Design review of the part built by this model. Coordinates are the model's own, in mm. Face numbers are marked on the shaded views. Coordinates: 2 decimals unless noted, no trailing zeros. Loops run counter-clockwise (first coordinate to the right, second up) from the corner with the lowest first, then second, coordinate; pieces in that order, holes last. Notation, with made-up numbers: (69, 0) -> (99, 0) arc R18 ccw to (99, 25) -> close; hole circle Ø1 at (21.5, 10). An arc over 180 degrees is marked (long way). Answer as a JSON object with one key per item and string values.
```python
from build123d import *

# Parameters (mm, degrees)
BASIS_BLECH1_DEPTH              = 57.5
SCHNITT_LINEAR_AUSTRAGEN1_REACH = 68.785
SKIZZE6_R                       = 4
SKIZZE6_R_2                     = 1.2
SCHNITT_LINEAR_AUSTRAGEN2_REACH = 68.785
SKIZZE7_R                       = 1.65


# Sheet-metal steps are written as plain solids
with BuildPart() as part:
    # Skizze1 → Basis-Blech1 (new, symmetric)
    with BuildSketch(Plane(origin=(0, 0, 0), x_dir=(0, 0, -1), z_dir=(1, 0, 0))):
        with BuildLine():
            Line((-10.5, 25), (-10.5, 0.2))
            ThreePointArc((-10.5, 0.2), (-10.441421356, 0.058578644), (-10.3, 0))
            Line((-10.3, 0), (10.3, 0))
            ThreePointArc((10.3, 0), (10.441421356, 0.058578644), (10.5, 0.2))
            Line((10.5, 0.2), (10.5, 19))
            Line((10.5, 19), (11.5, 19))
            Line((11.5, 19), (11.5, 0.2))
            ThreePointArc((11.5, 0.2), (11.148528137, -0.648528137), (10.3, -1))
            Line((10.3, -1), (-10.3, -1))
            ThreePointArc((-10.3, -1), (-11.148528137, -0.648528137), (-11.5, 0.2))
            Line((-11.5, 0.2), (-11.5, 25))
            Line((-11.5, 25), (-10.5, 25))
        make_face()
    extrude(amount=BASIS_BLECH1_DEPTH, both=True)

    # Skizze6 → Schnitt-Linear austragen1 (cut, up to next)
    with BuildSketch(Plane.XY.offset(11.5), mode=Mode.PRIVATE) as schnitt_linear_austragen1_sk1:
        with Locations((-40, 12)):
            Circle(SKIZZE6_R)
    schnitt_linear_austragen1_tool1 = extrude(schnitt_linear_austragen1_sk1.sketch, amount=-SCHNITT_LINEAR_AUSTRAGEN1_REACH, mode=Mode.PRIVATE) & part.part
    # Skizze6 → Schnitt-Linear austragen1 (cut, up to next)
    with BuildSketch(Plane.XY.offset(11.5), mode=Mode.PRIVATE) as schnitt_linear_austragen1_sk2:
        with Locations((-53, 15)):
            Circle(SKIZZE6_R_2)
    schnitt_linear_austragen1_tool2 = extrude(schnitt_linear_austragen1_sk2.sketch, amount=-SCHNITT_LINEAR_AUSTRAGEN1_REACH, mode=Mode.PRIVATE) & part.part
    # Skizze6 → Schnitt-Linear austragen1 (cut, up to next)
    with BuildSketch(Plane.XY.offset(11.5), mode=Mode.PRIVATE) as schnitt_linear_austragen1_sk3:
        with Locations((-53, 3)):
            Circle(SKIZZE6_R_2)
    schnitt_linear_austragen1_tool3 = extrude(schnitt_linear_austragen1_sk3.sketch, amount=-SCHNITT_LINEAR_AUSTRAGEN1_REACH, mode=Mode.PRIVATE) & part.part
    # Skizze6 → Schnitt-Linear austragen1 (cut, up to next)
    with BuildSketch(Plane.XY.offset(11.5), mode=Mode.PRIVATE) as schnitt_linear_austragen1_sk4:
        with Locations((-27, 15)):
            Circle(SKIZZE6_R_2)
    schnitt_linear_austragen1_tool4 = extrude(schnitt_linear_austragen1_sk4.sketch, amount=-SCHNITT_LINEAR_AUSTRAGEN1_REACH, mode=Mode.PRIVATE) & part.part
    # Skizze6 → Schnitt-Linear austragen1 (cut, up to next)
    with BuildSketch(Plane.XY.offset(11.5), mode=Mode.PRIVATE) as schnitt_linear_austragen1_sk5:
        with Locations((-27, 3)):
            Circle(SKIZZE6_R_2)
    schnitt_linear_austragen1_tool5 = extrude(schnitt_linear_austragen1_sk5.sketch, amount=-SCHNITT_LINEAR_AUSTRAGEN1_REACH, mode=Mode.PRIVATE) & part.part
    # Skizze6 → Schnitt-Linear austragen1 (cut, up to next)
    with BuildSketch(Plane.XY.offset(11.5), mode=Mode.PRIVATE) as schnitt_linear_austragen1_sk6:
        with Locations(Location((53, 3, 0), (0, 0, 90))):
            Circle(SKIZZE6_R_2)
    schnitt_linear_austragen1_tool6 = extrude(schnitt_linear_austragen1_sk6.sketch, amount=-SCHNITT_LINEAR_AUSTRAGEN1_REACH, mode=Mode.PRIVATE) & part.part
    # Skizze6 → Schnitt-Linear austragen1 (cut, up to next)
    with BuildSketch(Plane.XY.offset(11.5), mode=Mode.PRIVATE) as schnitt_linear_austragen1_sk7:
        with Locations(Location((27, 3, 0), (0, 0, 90))):
            Circle(SKIZZE6_R_2)
    schnitt_linear_austragen1_tool7 = extrude(schnitt_linear_austragen1_sk7.sketch, amount=-SCHNITT_LINEAR_AUSTRAGEN1_REACH, mode=Mode.PRIVATE) & part.part
    # Skizze6 → Schnitt-Linear austragen1 (cut, up to next)
    with BuildSketch(Plane.XY.offset(11.5), mode=Mode.PRIVATE) as schnitt_linear_austragen1_sk8:
        with Locations(Location((27, 15, 0), (0, 0, 90))):
            Circle(SKIZZE6_R_2)
    schnitt_linear_austragen1_tool8 = extrude(schnitt_linear_austragen1_sk8.sketch, amount=-SCHNITT_LINEAR_AUSTRAGEN1_REACH, mode=Mode.PRIVATE) & part.part
    # Skizze6 → Schnitt-Linear austragen1 (cut, up to next)
    with BuildSketch(Plane.XY.offset(11.5), mode=Mode.PRIVATE) as schnitt_linear_austragen1_sk9:
        with Locations(Location((40, 12, 0), (0, 0, 90))):
            Circle(SKIZZE6_R)
    schnitt_linear_austragen1_tool9 = extrude(schnitt_linear_austragen1_sk9.sketch, amount=-SCHNITT_LINEAR_AUSTRAGEN1_REACH, mode=Mode.PRIVATE) & part.part
    # Skizze6 → Schnitt-Linear austragen1 (cut, up to next)
    with BuildSketch(Plane.XY.offset(11.5), mode=Mode.PRIVATE) as schnitt_linear_austragen1_sk10:
        with Locations(Location((53, 15, 0), (0, 0, 90))):
            Circle(SKIZZE6_R_2)
    schnitt_linear_austragen1_tool10 = extrude(schnitt_linear_austragen1_sk10.sketch, amount=-SCHNITT_LINEAR_AUSTRAGEN1_REACH, mode=Mode.PRIVATE) & part.part
    # Skizze6 → Schnitt-Linear austragen1 (cut, up to next)
    with BuildSketch(Plane.XY.offset(11.5), mode=Mode.PRIVATE) as schnitt_linear_austragen1_sk11:
        with BuildLine():
            Line((-20, 16), (-10, 16))
            ThreePointArc((-10, 16), (-6, 12), (-10, 8))
            Line((-10, 8), (-20, 8))
            ThreePointArc((-20, 8), (-24, 12), (-20, 16))
        make_face()
    schnitt_linear_austragen1_tool11 = extrude(schnitt_linear_austragen1_sk11.sketch, amount=-SCHNITT_LINEAR_AUSTRAGEN1_REACH, mode=Mode.PRIVATE) & part.part
    # Skizze6 → Schnitt-Linear austragen1 (cut, up to next)
    with BuildSketch(Plane.XY.offset(11.5), mode=Mode.PRIVATE) as schnitt_linear_austragen1_sk12:
        with BuildLine():
            Line((20, 16), (10, 16))
            ThreePointArc((10, 16), (6, 12), (10, 8))
            Line((10, 8), (20, 8))
            ThreePointArc((20, 8), (24, 12), (20, 16))
        make_face()
    schnitt_linear_austragen1_tool12 = extrude(schnitt_linear_austragen1_sk12.sketch, amount=-SCHNITT_LINEAR_AUSTRAGEN1_REACH, mode=Mode.PRIVATE) & part.part
    add(schnitt_linear_austragen1_tool1.solids().sort_by_distance((-40, 12, 11.5))[0], mode=Mode.SUBTRACT)
    add(schnitt_linear_austragen1_tool2.solids().sort_by_distance((-53, 15, 11.5))[0], mode=Mode.SUBTRACT)
    add(schnitt_linear_austragen1_tool3.solids().sort_by_distance((-53, 3, 11.5))[0], mode=Mode.SUBTRACT)
    add(schnitt_linear_austragen1_tool4.solids().sort_by_distance((-27, 15, 11.5))[0], mode=Mode.SUBTRACT)
    add(schnitt_linear_austragen1_tool5.solids().sort_by_distance((-27, 3, 11.5))[0], mode=Mode.SUBTRACT)
    add(schnitt_linear_austragen1_tool6.solids().sort_by_distance((53, 3, 11.5))[0], mode=Mode.SUBTRACT)
    add(schnitt_linear_austragen1_tool7.solids().sort_by_distance((27, 3, 11.5))[0], mode=Mode.SUBTRACT)
    add(schnitt_linear_austragen1_tool8.solids().sort_by_distance((27, 15, 11.5))[0], mode=Mode.SUBTRACT)
    add(schnitt_linear_austragen1_tool9.solids().sort_by_distance((40, 12, 11.5))[0], mode=Mode.SUBTRACT)
    add(schnitt_linear_austragen1_tool10.solids().sort_by_distance((53, 15, 11.5))[0], mode=Mode.SUBTRACT)
    add(schnitt_linear_austragen1_tool11.solids().sort_by_distance((-15, 12, 11.5))[0], mode=Mode.SUBTRACT)
    add(schnitt_linear_austragen1_tool12.solids().sort_by_distance((15, 12, 11.5))[0], mode=Mode.SUBTRACT)

    # Skizze7 → Schnitt-Linear austragen2 (cut, up to next)
    with BuildSketch(Plane(origin=(0, 0, -11.5), x_dir=(-1, 0, 0), z_dir=(0, 0, -1)), mode=Mode.PRIVATE) as schnitt_linear_austragen2_sk1:
        with Locations(Location((-40, 11.5, 0), (0, 0, 90))):
            Circle(SKIZZE7_R)
    schnitt_linear_austragen2_tool1 = extrude(schnitt_linear_austragen2_sk1.sketch, amount=-SCHNITT_LINEAR_AUSTRAGEN2_REACH, mode=Mode.PRIVATE) & part.part
    # Skizze7 → Schnitt-Linear austragen2 (cut, up to next)
    with BuildSketch(Plane(origin=(0, 0, -11.5), x_dir=(-1, 0, 0), z_dir=(0, 0, -1)), mode=Mode.PRIVATE) as schnitt_linear_austragen2_sk2:
        with Locations(Location((-20, 11.5, 0), (0, 0, 90))):
            Circle(SKIZZE7_R)
    schnitt_linear_austragen2_tool2 = extrude(schnitt_linear_austragen2_sk2.sketch, amount=-SCHNITT_LINEAR_AUSTRAGEN2_REACH, mode=Mode.PRIVATE) & part.part
    # Skizze7 → Schnitt-Linear austragen2 (cut, up to next)
    with BuildSketch(Plane(origin=(0, 0, -11.5), x_dir=(-1, 0, 0), z_dir=(0, 0, -1)), mode=Mode.PRIVATE) as schnitt_linear_austragen2_sk3:
        with Locations(Location((-10, 11.5, 0), (0, 0, 90))):
            Circle(SKIZZE7_R)
    schnitt_linear_austragen2_tool3 = extrude(schnitt_linear_austragen2_sk3.sketch, amount=-SCHNITT_LINEAR_AUSTRAGEN2_REACH, mode=Mode.PRIVATE) & part.part
    # Skizze7 → Schnitt-Linear austragen2 (cut, up to next)
    with BuildSketch(Plane(origin=(0, 0, -11.5), x_dir=(-1, 0, 0), z_dir=(0, 0, -1)), mode=Mode.PRIVATE) as schnitt_linear_austragen2_sk4:
        with Locations(Location((10, 11.5, 0), (0, 0, 90))):
            Circle(SKIZZE7_R)
    schnitt_linear_austragen2_tool4 = extrude(schnitt_linear_austragen2_sk4.sketch, amount=-SCHNITT_LINEAR_AUSTRAGEN2_REACH, mode=Mode.PRIVATE) & part.part
    # Skizze7 → Schnitt-Linear austragen2 (cut, up to next)
    with BuildSketch(Plane(origin=(0, 0, -11.5), x_dir=(-1, 0, 0), z_dir=(0, 0, -1)), mode=Mode.PRIVATE) as schnitt_linear_austragen2_sk5:
        with Locations(Location((20, 11.5, 0), (0, 0, 90))):
            Circle(SKIZZE7_R)
    schnitt_linear_austragen2_tool5 = extrude(schnitt_linear_austragen2_sk5.sketch, amount=-SCHNITT_LINEAR_AUSTRAGEN2_REACH, mode=Mode.PRIVATE) & part.part
    # Skizze7 → Schnitt-Linear austragen2 (cut, up to next)
    with BuildSketch(Plane(origin=(0, 0, -11.5), x_dir=(-1, 0, 0), z_dir=(0, 0, -1)), mode=Mode.PRIVATE) as schnitt_linear_austragen2_sk6:
        with Locations(Location((40, 11.5, 0), (0, 0, 90))):
            Circle(SKIZZE7_R)
    schnitt_linear_austragen2_tool6 = extrude(schnitt_linear_austragen2_sk6.sketch, amount=-SCHNITT_LINEAR_AUSTRAGEN2_REACH, mode=Mode.PRIVATE) & part.part
    add(schnitt_linear_austragen2_tool1.solids().sort_by_distance((40, 11.5, -11.5))[0], mode=Mode.SUBTRACT)
    add(schnitt_linear_austragen2_tool2.solids().sort_by_distance((20, 11.5, -11.5))[0], mode=Mode.SUBTRACT)
    add(schnitt_linear_austragen2_tool3.solids().sort_by_distance((10, 11.5, -11.5))[0], mode=Mode.SUBTRACT)
    add(schnitt_linear_austragen2_tool4.solids().sort_by_distance((-10, 11.5, -11.5))[0], mode=Mode.SUBTRACT)
    add(schnitt_linear_austragen2_tool5.solids().sort_by_distance((-20, 11.5, -11.5))[0], mode=Mode.SUBTRACT)
    add(schnitt_linear_austragen2_tool6.solids().sort_by_distance((-40, 11.5, -11.5))[0], mode=Mode.SUBTRACT)


solid = part.part
```
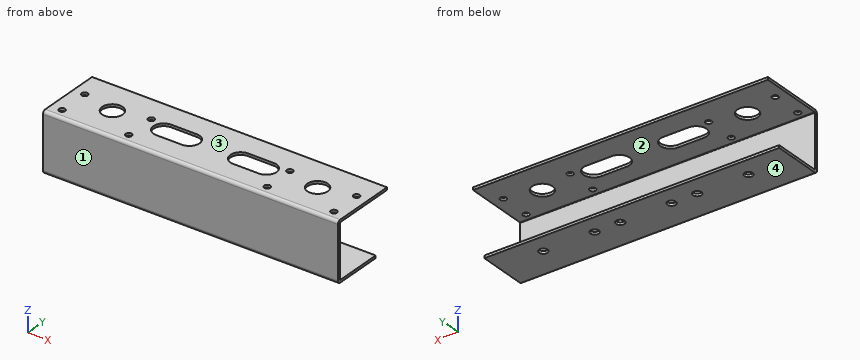
1) Wall thickness on probe 1 along Z at (x, y) = (29, 7.5); probe 2 along Y at (x, z) = (53, 11.2); probe 3 along Z at (x, y) = (9, 23.75): over which ranges is each line inside the solid? List them lowest first.
Completed:
{"probe 1": "-11.5 to -10.5, 10.5 to 11.5", "probe 2": "-0.59 to 1.8, 4.2 to 13.8, 16.2 to 25", "probe 3": "10.5 to 11.5"}
2) Add section D-D, the plane y = 21.25. Give the boundary of the cut face in (x, z).
Completed:
{"outline": "(-57.5, 10.5) -> (57.5, 10.5) -> (57.5, 11.5) -> (-57.5, 11.5) -> close"}
3) Add section B-B, the plane y = 3. Give the boundary of the cut face in (x, z).
Completed:
{"outline": "(-57.5, -11.5) -> (57.5, -11.5) -> (57.5, -10.5) -> (-57.5, -10.5) -> close; (-57.5, 10.5) -> (-54.2, 10.5) -> (-54.2, 11.5) -> (-57.5, 11.5) -> close; (-51.8, 10.5) -> (-28.2, 10.5) -> (-28.2, 11.5) -> (-51.8, 11.5) -> close; (-25.8, 10.5) -> (25.8, 10.5) -> (25.8, 11.5) -> (-25.8, 11.5) -> close; (28.2, 10.5) -> (51.8, 10.5) -> (51.8, 11.5) -> (28.2, 11.5) -> close; (54.2, 10.5) -> (57.5, 10.5) -> (57.5, 11.5) -> (54.2, 11.5) -> close"}
4) The part is to be moulded in two halves that separate along Z. For the marked faces 1, 2, 3 and 4, say which applies: pulls with the +Z half, pulls with the -Z half, needs draft (parallel to the pull), parting line crosses it, or undercut.
Completed:
{"face 1": "needs draft", "face 2": "undercut", "face 3": "pulls with the +Z half", "face 4": "pulls with the -Z half"}
5) Clearance check with flat-ended pins moving along their axes: pin 1 Ø1.5 at (x, z) = (10.5, 9) entering from +Y; pin 2 Ø2 at (x, y) = (-53, 15) entering from +Z. State where each tip first meets the part, or that it passes through.
Completed:
{"pin 1": "y = 0", "pin 2": "z = -10.5"}
6) Add section C-C, the plane x = 27. Give the boundary of the cut face in (y, z), and give its area (3 significant figures).
Completed:
{"outline": "(-1, -10.3) arc R1.2 ccw to (0.2, -11.5) -> (19, -11.5) -> (19, -10.5) -> (0.2, -10.5) arc R0.2 cw to (0, -10.3) -> (0, 10.3) arc R0.2 cw to (0.2, 10.5) -> (1.8, 10.5) -> (1.8, 11.5) -> (0.2, 11.5) arc R1.2 ccw to (-1, 10.3) -> close; (4.2, 10.5) -> (13.8, 10.5) -> (13.8, 11.5) -> (4.2, 11.5) -> close; (16.2, 10.5) -> (25, 10.5) -> (25, 11.5) -> (16.2, 11.5) -> close", "area": "61.6 mm²"}
7) Add section A-A, the plane x = -40. Give the boundary of the cut face in (y, z), and give its area (3 significant figures).
Completed:
{"outline": "(-1, -10.3) arc R1.2 ccw to (0.2, -11.5) -> (9.85, -11.5) -> (9.85, -10.5) -> (0.2, -10.5) arc R0.2 cw to (0, -10.3) -> (0, 10.3) arc R0.2 cw to (0.2, 10.5) -> (8, 10.5) -> (8, 11.5) -> (0.2, 11.5) arc R1.2 ccw to (-1, 10.3) -> close; (13.15, -11.5) -> (19, -11.5) -> (19, -10.5) -> (13.15, -10.5) -> close; (16, 10.5) -> (25, 10.5) -> (25, 11.5) -> (16, 11.5) -> close", "area": "55.1 mm²"}
